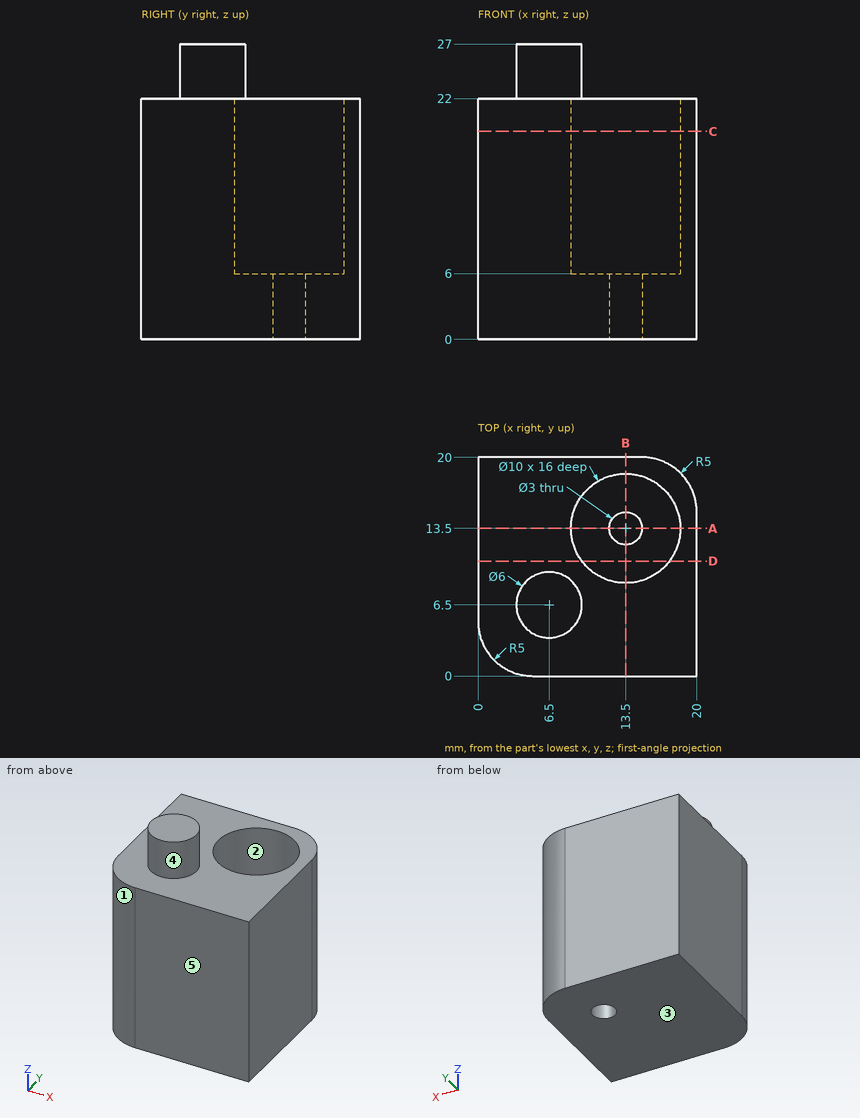
Print and shaded views of the part. All mm, measured from the part's lowest x, y and z. A direction names the side the tool comes from. Coordinates: 2 decimals unless noted, no trailing zeros. Order: outer loops, then holes, each group sorted by start corner. A loop starts at its lowest first (then second) coordinate and runs counter-clockwise, first axis right, second up.
(1) Slice it at D-D, the plane y = 10.5. Write the cut outline in (x, z).
Check sheet entries:
outline: (0, 0) - (20, 0) - (20, 22) - (17.5, 22) - (17.5, 6) - (9.5, 6) - (9.5, 22) - (0, 22) - close
(2) Pull direction X, two halves, no side cores. Call the marked faces 1, 2 and 3: pulls with the +X half, pulls with the -X half, needs draft (parallel to the pull), parting line crosses it, or undercut.
Check sheet entries:
face 1: pulls with the -X half
face 2: undercut
face 3: needs draft
(3) Slice it at A-A, the plane y = 13.5. Write the cut outline in (x, z).
Check sheet entries:
outline: (0, 0) - (12, 0) - (12, 6) - (8.5, 6) - (8.5, 22) - (0, 22) - close; (15, 0) - (20, 0) - (20, 22) - (18.5, 22) - (18.5, 6) - (15, 6) - close
(4) Tool access for the marked faces 4 and 5: list every direction of +Z, -Z, +X, -X, +Y, -Y with a clear straight run to the whole face (end or side of a thin tool).
Check sheet entries:
face 4: +Z
face 5: +Z, -Z, +X, -X, -Y
(5) Probe L1, parallel to Y at x = 13.5, z = 3.8; L2, parallel to Y at x = 13.5, z = 12.5. List the from-to ranges inside material, lowest first.
Check sheet entries:
L1: y = 0 to 12, 15 to 20
L2: y = 0 to 8.5, 18.5 to 20
(6) Slice it at C-C, the plane z = 19. Write the cut outline in (x, y).
Check sheet entries:
outline: (0, 5) arc R5 ccw to (5, 0) - (20, 0) - (20, 15) arc R5 ccw to (15, 20) - (0, 20) - close; hole circle Ø10 at (13.5, 13.5)
